Part model, mm, in its own coordinate system. A direction names the side the tool comes from. Coordinates: 2 decimals unless noted, no trailing zeros. Loops run counter-clockwise (first coordinate to the right, second up) from the corner with the lowest first, then second, coordinate; pieces in that order, holes last. Notation, with made-up numbers: M -28.75,78.5 L 28.25,78.5 A17 cw 28.25,97.5 Z; hole C 7.5,-12.5 d5. An arc over 180 degrees is marked long. Answer as a JSON object with one key per item and string values. Group by question number.
1. Drop flat-ended pins along their axis: pin 1 Ø4.5 at (x, y) = (0, 0) entering from -Z; pin 2 Ø1.5 at (y, z) = (11.5, -1) entering from -X; pin 3 Ø6 at (x, y) = (0, 2) entering from +Z (3 decimals); pin 4 Ø1 at (x, z) = (-0.5, -2) entering from +Y. Give the stop position or say it passes through.
2. Saw through at B-B on z = -2.1. Count the separate pieces of the cut face and the enclosed holes in it, then the cut area to 3 significant figures.
3. 3-axis set-ups, long thin cutter, end or side, ignore diameter. For faces 4 (the face through (0, 6.096, -2)), 5 (the face through (0, -6, -4.699)), 6 (the face through (-22.131, -8.414, -2.382)): which of +Z, -Z, +X, -X, +Y, -Y reach the whole face in a straight line?
4. Saw through at A-A on x = 0. Write the cut outline in (y, z) (1 decimal).
5. Drill centre lines: L1, parallel to X at y = -8, z = -3.55; L2, parallel to Y at x = 1, z = -2.05; L3, parallel to X at y = -5, z = -4.1. Where is each one in solid material? Low to high.
6. Mould opens along X. For faces 1 (the face through (27.276, -11.309, -4.313)), 2 (the face through (-7.833, -7.192, -2.382)), 3 (the face through (-6, -6, 0)) say: released by +X, released by -X, zero draft, split by the parting line, or undercut.
from build123d import *

# Parameters (mm, degrees)
SKETCH1_R           = 9.525
BOSS_EXTRUDE1_DEPTH = 4.699
CUT_EXTRUDE1_DEPTH  = 3.175
SKETCH5_R           = 2.032
CUT_EXTRUDE2_DEPTH  = 43.021745862
FILLET1_R           = 5.08


with BuildPart() as part:
    # Sketch1 → Boss-Extrude1 (new body)
    with BuildSketch(Plane.XY):
        with BuildLine():
            ThreePointArc((1.5875, 25.350342083), (0, 25.4), (-1.5875, 25.350342083))
            Line((-1.5875, 25.350342083), (-1.5875, 9.391776656))
            ThreePointArc((-1.5875, 9.391776656), (0, 9.525), (1.5875, 9.391776656))
            Line((1.5875, 9.391776656), (1.5875, 25.350342083))
        make_face()
        Circle(SKETCH1_R)
        with BuildLine():
            ThreePointArc((21.160290239, -14.04998637), (21.997045256, -12.7), (22.747790239, -11.300355713))
            Line((22.747790239, -11.300355713), (8.92726717, -3.321072999))
            ThreePointArc((8.92726717, -3.321072999), (8.248891971, -4.7625), (7.33976717, -6.070703656))
            Line((7.33976717, -6.070703656), (21.160290239, -14.04998637))
        make_face()
        with BuildLine():
            Line((-8.92726717, -3.321072999), (-22.747790239, -11.300355713))
            ThreePointArc((-22.747790239, -11.300355713), (-21.997045256, -12.7), (-21.160290239, -14.04998637))
            Line((-21.160290239, -14.04998637), (-7.33976717, -6.070703656))
            ThreePointArc((-7.33976717, -6.070703656), (-8.248891971, -4.7625), (-8.92726717, -3.321072999))
        make_face()
    extrude(amount=-BOSS_EXTRUDE1_DEPTH)

    # Sweep1: sweep along a path in Sketch4
    with BuildLine(Plane.XY) as sweep1_path:
        CenterArc((0, 0), 25.4, 0, 360)
    # Sketch3 → Sweep1 (sweep)
    with BuildSketch(Plane(origin=(0, 0, 0), x_dir=(0, 0, -1), z_dir=(1, 0, 0))):
        with BuildLine():
            Line((0, 25.4), (0, 29.5275))
            Line((0, 29.5275), (0.762, 29.5275))
            ThreePointArc((0.762, 29.5275), (2.3495, 27.94), (3.937, 29.5275))
            Line((3.937, 29.5275), (4.699, 29.5275))
            Line((4.699, 29.5275), (4.699, 25.4))
            Line((4.699, 25.4), (0, 25.4))
        make_face()
    sweep(path=sweep1_path.line)

    # Sketch2 → Cut-Extrude1 (cut)
    with BuildSketch(Plane.XY):
        Polygon((7.039054482, 0), (3.519527241, 6.096), (-3.519527241, 6.096), (-7.039054482, 0), (-3.519527241, -6.096), (3.519527241, -6.096), align=None)
    extrude(amount=-CUT_EXTRUDE1_DEPTH, mode=Mode.SUBTRACT)

    # Sketch5 → Cut-Extrude2 (cut, through all)
    with BuildSketch(Plane.XY):
        Circle(SKETCH5_R)
    extrude(amount=-CUT_EXTRUDE2_DEPTH, mode=Mode.SUBTRACT)

    # Fillet1
    fillet1_edges = [part.edges().sort_by_distance(p)[0] for p in [
        (-1.5875, 25.350342083, -2.3495),
        (1.5875, 25.350342083, -2.3495),
        (1.5875, 9.391776656, -2.3495),
        (8.92726717, -3.321072999, -2.3495),
        (22.747790239, -11.300355713, -2.3495),
        (21.160290239, -14.04998637, -2.3495),
        (-7.33976717, -6.070703656, -2.3495),
        (-21.160290239, -14.04998637, -2.3495),
        (-22.747790239, -11.300355713, -2.3495),
        (-8.92726717, -3.321072999, -2.3495),
        (-1.5875, 9.391776656, -2.3495),
    ]]
    fillet(fillet1_edges, radius=FILLET1_R)


solid = part.part
Outcome:
{
 "1": {"pin 1": "stops at z = -4.7", "pin 2": "stops at x = -27.49", "pin 3": "stops at z = -3.175", "pin 4": "stops at y = 28.18"},
 "2": {"separate pieces": "1", "enclosed holes": "4", "area": "804 mm²"},
 "3": {"face 4": "+Z", "face 5": "-Z, +X, -X, +Y, -Y", "face 6": "+Z, -Z"},
 "4": {"outline": "M -29.5,-4.7 L -25.4,-4.7 L -25.4,0 L -29.5,0 L -29.5,-0.8 A1.6 cw -29.5,-3.9 Z; M -9.5,-4.7 L -2,-4.7 L -2,-3.2 L -6.1,-3.2 L -6.1,0 L -9.5,0 Z; M 2,-4.7 L 29.5,-4.7 L 29.5,-3.9 A1.6 cw 29.5,-0.8 L 29.5,0 L 6.1,0 L 6.1,-3.2 L 2,-3.2 Z"},
 "5": {"L1": "x = -27.34 to -22.85, -17.03 to -10.68, -5.17 to 5.17, 10.68 to 17.03, 22.85 to 27.34", "L2": "y = -27.95 to -25.38, -9.47 to -6.1, 6.1 to 27.95", "L3": "x = -29.1 to -24.9, -11.85 to 11.85, 24.9 to 29.1"},
 "6": {"face 1": "split by the parting line", "face 2": "undercut", "face 3": "zero draft"}
}
